Read the model definition and answer for the solid it produces. Units are mm, in the model's axes. Round coordinates to 2 decimals unless told otherwise and drop trailing zeros. Order: outer loops, then holes, each group sorted by start corner. A loop starts at its lowest first (then second) coordinate and runs counter-clockwise, first axis right, second up. Notation, with made-up numbers: (76, -39.5) -> (130, -39.5) arc R10 cw to (130, -29.5) -> close; hole circle Ø7 at (-5.75, 3). An arc over 180 degrees is marked (long way). Use a Markdown table: item, result. Add a question column.
1. Section A-A, the plane x = 2.5 is taken. Give the vertices of the cut face in (y, z), then the cut area to 3 significant figures.
2. Given pin 1 (1.4 mm diameter, centred on x = 39.5, z = 0, fed in from -Y); pin 2 (1.1 mm diameter, centred on y = -2.5, z = -1, fed in from +X); pin 3 (1.4 mm diameter, centred on x = -3, y = -3, fed in from +Z), each flat-ended and moving along its own axis, determine where each tip first touches the part or whether it passes through.
3. Section B-B, the plane z = 1 is taken. Give the vertices of the cut face in (x, y), then the cut area to 3 significant figures.
4. Consider L1, parallel to Z at x = 31.5, y = -4.05; L2, parallel to X at y = -3.9, z = 9; L3, parallel to X at y = -1.1, z = -1.25. Determine where each line is inside the solid, lowest interval first. Write a range as [from, to].
5. Section C-C, the plane z = -8.5 is taken. Give the vertices of the cut face in (x, y), then the cut area to 3 significant figures.
```python
from build123d import *

# Parameters (mm, degrees)
SKETCH1_W           = 80
SKETCH1_H           = 25
BOSS_EXTRUDE1_DEPTH = 1.75
SKETCH2_W           = 77.5
SKETCH2_H           = 21
BOSS_EXTRUDE3_DEPTH = 2.75
CAVITY1_START       = -40
CAVITY1_OUTLINE_W   = 1.75
CAVITY1_OUTLINE_H   = 25
CAVITY1_DEPTH       = 80
CAVITY1_START_2     = -5
CAVITY1_2_DEPTH     = 10
CUT_EXTRUDE1_START  = -0.4
CUT_EXTRUDE1_DEPTH  = 10.8
SKETCH5_W           = 80
SKETCH5_H           = 24
BOSS_EXTRUDE4_DEPTH = 1.75
SKETCH7_W           = 1.25
SKETCH7_H           = 15
CUT_EXTRUDE2_DEPTH  = 1
SKETCH8_W           = 1.25
SKETCH8_H           = 15
BOSS_EXTRUDE5_DEPTH = 1


# Read off the part's stored shape, not the designer's step: Cavity1
with BuildPart() as part:
    # Sketch1 → Boss-Extrude1 (new body)
    with BuildSketch(Plane(origin=(0, 0, 0), x_dir=(1, 0, 0), z_dir=(0, 1, 0))):
        Rectangle(SKETCH1_W, SKETCH1_H)
    extrude(amount=-BOSS_EXTRUDE1_DEPTH)

    # Sketch2 → Boss-Extrude3 (add)
    with BuildSketch(Plane(origin=(0, -1.75, 0), x_dir=(-1, 0, 0), z_dir=(0, -1, 0))):
        Rectangle(SKETCH2_W, SKETCH2_H)
    extrude(amount=BOSS_EXTRUDE3_DEPTH)

    # Cavity1 outline → Cavity1 (cut)
    with BuildSketch(Plane.YZ.offset(CAVITY1_START)):
        with Locations((-0.875, 0)):
            Rectangle(CAVITY1_OUTLINE_W, CAVITY1_OUTLINE_H)
    extrude(amount=CAVITY1_DEPTH, mode=Mode.SUBTRACT)

    # Cavity1 2 outline → Cavity1 2 (cut)
    with BuildSketch(Plane.YZ.offset(CAVITY1_START_2)):
        with BuildLine():
            Line((-2.717157288, 10.282842712), (-2.5, 10.5))
            Line((-2.5, 10.5), (-3.5, 10.5))
            Line((-3.5, 10.5), (-3.282842712, 10.282842712))
            ThreePointArc((-3.282842712, 10.282842712), (-3, 10.165685425), (-2.717157288, 10.282842712))
        make_face()
        with BuildLine():
            Line((-3.5, -10.5), (-2.5, -10.5))
            Line((-2.5, -10.5), (-2.717157288, -10.282842712))
            ThreePointArc((-2.717157288, -10.282842712), (-3, -10.165685425), (-3.282842712, -10.282842712))
            Line((-3.282842712, -10.282842712), (-3.5, -10.5))
        make_face()
    extrude(amount=CAVITY1_2_DEPTH, mode=Mode.SUBTRACT)

    # Sketch4 → Cut-Extrude1 (cut)
    with BuildSketch(Plane(origin=(-5, 0, 0), x_dir=(0, 0, -1), z_dir=(1, 0, 0)).offset(CUT_EXTRUDE1_START)):
        Polygon((-10.800137225, -1.63417735), (-9.57584768, -2.858466895), (-10.943501518, -4.226511252), align=None)
    cut_extrude1 = extrude(amount=CUT_EXTRUDE1_DEPTH, mode=Mode.SUBTRACT)

    # Mirror1: Cut-Extrude1 across plane
    add(cut_extrude1.mirror(Plane.XY), mode=Mode.SUBTRACT)

    # Sketch5 → Boss-Extrude4 (add)
    with BuildSketch(Plane(origin=(0, -1.75, 0), x_dir=(1, 0, 0), z_dir=(0, 1, 0))):
        Rectangle(SKETCH5_W, SKETCH5_H)
    extrude(amount=BOSS_EXTRUDE4_DEPTH)

    # Sketch7 → Cut-Extrude2 (cut)
    with BuildSketch(Plane.XZ.offset(1.75)):
        with Locations((-39.375, 0)):
            Rectangle(SKETCH7_W, SKETCH7_H)
    cut_extrude2 = extrude(amount=-CUT_EXTRUDE2_DEPTH, mode=Mode.SUBTRACT)

    # Mirror2: Cut-Extrude2 across plane
    add(cut_extrude2.mirror(Plane(origin=(0, 0, 0), x_dir=(0, 0, 1), z_dir=(1, 0, 0))), mode=Mode.SUBTRACT)

    # Sketch8 → Boss-Extrude5 (add)
    with BuildSketch(Plane(origin=(0, -0.75, 0), x_dir=(-1, 0, 0), z_dir=(0, -1, 0))):
        with Locations((39.375, 0)):
            Rectangle(SKETCH8_W, SKETCH8_H)
    extrude(amount=BOSS_EXTRUDE5_DEPTH)


solid = part.part
```
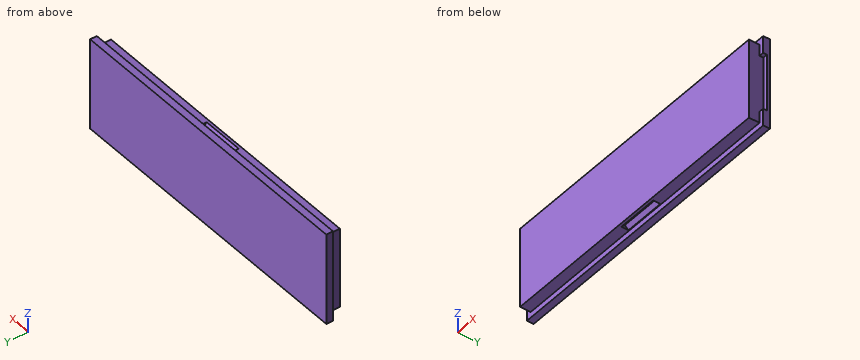
Verdict:
| question | item | result |
|---|---|---|
| 1 | outline | (-4.5, -10.5) -> (-3.78, -10.5) -> (-2.86, -9.58) -> (-1.93, -10.5) -> (-1.75, -10.5) -> (-1.75, -12) -> (0, -12) -> (0, 12) -> (-1.75, 12) -> (-1.75, 10.5) -> (-1.93, 10.5) -> (-2.86, 9.58) -> (-3.78, 10.5) -> (-4.5, 10.5) -> close |
| 1 | area | 98.0 mm2 |
| 2 | pin 1 | stops at y = -0.75 |
| 2 | pin 2 | stops at x = 38.75 |
| 2 | pin 3 | stops at z = 10.42 |
| 3 | outline | (-40, -1.75) -> (-38.75, -1.75) -> (-38.75, -4.5) -> (38.75, -4.5) -> (38.75, -0.75) -> (40, -0.75) -> (40, 0) -> (-40, 0) -> close |
| 3 | area | 352 mm2 |
| 4 | L1 | z = [-10.5, 10.5] |
| 4 | L2 | x = [-38.75, 38.75] |
| 4 | L3 | x = [-40, 38.75] |
| 5 | outline | (-40, -1.75) -> (-38.75, -1.75) -> (-38.75, -4.5) -> (38.75, -4.5) -> (38.75, -1.75) -> (40, -1.75) -> (40, 0) -> (-40, 0) -> close |
| 5 | area | 353 mm2 |
